Autodesk Inventor part; units mm, degrees
ref_plane "YZ Plane" through (0, 0, 0) normal (1, 0, 0) x (0, 1, 0)
ref_plane "XZ Plane" through (0, 0, 0) normal (0, 1, 0) x (-1, 0, 0)
ref_plane "XY Plane" through (0, 0, 0) normal (0, 0, 1) x (1, 0, 0)
sketch "Sketch1" plane through (0, 0, 0) normal (0, 0, 1) x (1, 0, 0)
  line L0 (0, 0) -> (76.2, 0)
  line L1 (76.2, 0) -> (76.2, 50.8)
  line L2 (76.2, 50.8) -> (0, 50.8)
  line L3 (0, 50.8) -> (0, 0)
  dimension "d0" = 76.2
  dimension "d1" = 50.8
extrude "Extrusion1" add sketch "Sketch1" along normal blind 76.2
shell "Shell1" thickness 4.7625 removed faces 4 at (50.8, 16.9333, 76.2) at (50.8, 50.8, 25.4) at (50.8, 16.9333, 0) at (0, 33.8667, 25.4)
sketch "Sketch3" plane through (0, 0, 0) normal (0, -1, 0) x (1, 0, 0)
  line L0 (64.6, 58.1) -> (11.6, 58.1) construction
  line L1 (11.6, 58.1) -> (11.6, 18.1) construction
  line L2 (11.6, 18.1) -> (64.6, 18.1) construction
  line L3 (64.6, 18.1) -> (64.6, 58.1) construction
  circle A0 centre (64.6, 18.1) radius 2.5
  circle A1 centre (64.6, 58.1) radius 2.5
  circle A2 centre (11.6, 58.1) radius 2.5
  circle A3 centre (11.6, 18.1) radius 2.5
  line L4 (76.2, 0) -> (76.2, 76.2) construction
  line L5 (0, 76.2) -> (76.2, 76.2) construction
  point P0 (0, 0)
  point P1 (64.6, 38.1)
  point P2 (76.2, 38.1)
  point P3 (38.1, 58.1)
  point P4 (38.1, 76.2)
  dimension "d6" = 40
  dimension "d7" = 53
  dimension "d8" = 5
  dimension "d16" = 0
extrude "Extrusion2" cut sketch "Sketch3" against normal blind 76.2
sketch "Sketch4" plane through (76.2, 0, 0) normal (1, 0, 0) x (0, 0, -1)
  circle A0 centre (-61.1, 32) radius 4
  circle A1 centre (-15.1, 32) radius 4
  line L0 (-61.1, 32) -> (-15.1, 32) construction
  line L1 (0, 0) -> (0, 50.8) construction
  line L2 (0, 50.8) -> (-76.2, 50.8) construction
  line L3 (-76.2, 0) -> (-76.2, 50.8) construction
  line L4 (0, 0) -> (-76.2, 0) construction
  point P0 (-38.1, 32)
  point P1 (0, 25.4)
  point P2 (-38.1, 50.8)
  dimension "d11" = 46
  dimension "d12" = 8
  dimension "d15" = 32
extrude "Extrusion3" cut sketch "Sketch4" against normal blind 76.2
fillet "Fillet1" radius 3.175 2 edges at (76.2, 0, 38.1) (71.4375, 4.7625, 38.1)
equation "\"BendRadius\" = Thickness"
equation "\"BendReliefWidth\" = Thickness"
equation "\"BendReliefDepth\" = 0.5 * Thickness"
equation "\"CornerReliefSize\" = 4 * Thickness"
equation "\"MinimumRemnant\" = 2 * Thickness"
equation "\"TransitionRadius\" = BendRadius"
equation "\"JacobiRadiusSize\" = BendRadius"
equation "\"GapSize\" = Thickness"
properties part number "2x3_L_Bracket"
The listing builds one solid part. Answer for the finished solid, in the listing's coordinates (mm). A direction names the side the tool comes from. Give positions to 0.01 mm unless a question says otherwise; leave off trailing zeros. Order: outer loops, then holes, each group sorted by start corner. A loop starts at its lowest first (then second) coordinate and runs counter-clockwise, first axis right, second up. Notation, with made-up numbers: (54, 35) - (86, 35) arc R8 cw to (86, 42) - close; hole circle Ø9 at (19, 53.25). An arc over 180 degrees is marked (long way). One line per item, written item: value. Start each with the question number.
1) The mould has two halves that part along X. Classify faces 1 (the face through (55, 3, 0)), 2 (the face through (75.25, 0.91, 38.63)), 3 (the face through (66.985, 2.348, 18.851)): released by +X, released by -X, zero draft, split by the parting line, or undercut.
2) A tool of negligible diameter and unlimited length cuts with its end or side. For faces 4 (the face through (74, 50.8, 38)), 5 (the face through (71.438, 29, 38)), from which of +Z, -Z, +X, -X, +Y, -Y can it reach the whole face along a straight path? Write none if from no direction.
3) Given pin 1 Ø10.5 at (y, z) = (32, 61.1) entering from +X; pin 2 Ø1.5 at (y, z) = (8, 57) entering from -X; pin 3 Ø1.5 at (x, z) = (37.5, 41.5) entering from +Y, each flat-ended and moving along its own axis, determine where each tip first touches the part or whether it passes through.
4) Find the intervals of material crossed by L1, parallel to Z at x = 64.6, y = 1.75; L2, parallel to X at y = 2, z = 58; L3, parallel to Y at x = 6.5, z = 15.5, in increasing order.
5) A cutting plane is placed at B-B on x = 64.6. Give the vertices of the cut face in (y, z).
6) A cutting plane is placed at A-A on y = 32. Give the vertices of the cut face in (x, z).
7) A cutting plane is placed at C-C on z = 58.1. State how many separate pieces and enclosed holes the cut face has, then the cut area to 3 significant figures.
Answer sheet:
1. face 1: zero draft
1. face 2: released by +X
1. face 3: undercut
2. face 4: +Z, -Z, +X, -X, +Y
2. face 5: +Z, -Z, -X, +Y
3. pin 1: stops at x = 76.2
3. pin 2: stops at x = 71.36
3. pin 3: stops at y = 4.76
4. L1: z = 0 to 15.6, 20.6 to 55.6, 60.6 to 76.2
4. L2: x = 0 to 9.1, 14.1 to 62.1, 67.1 to 75.97
4. L3: y = 0 to 4.76
5. outline: (0, 0) - (4.76, 0) - (4.76, 15.6) - (0, 15.6) - close; (0, 20.6) - (4.76, 20.6) - (4.76, 55.6) - (0, 55.6) - close; (0, 60.6) - (4.76, 60.6) - (4.76, 76.2) - (0, 76.2) - close
6. outline: (71.44, 0) - (76.2, 0) - (76.2, 11.1) - (71.44, 11.1) - close; (71.44, 19.1) - (76.2, 19.1) - (76.2, 57.1) - (71.44, 57.1) - close; (71.44, 65.1) - (76.2, 65.1) - (76.2, 76.2) - (71.44, 76.2) - close
7. separate pieces: 4
7. enclosed holes: 0
7. area: 509 mm2
